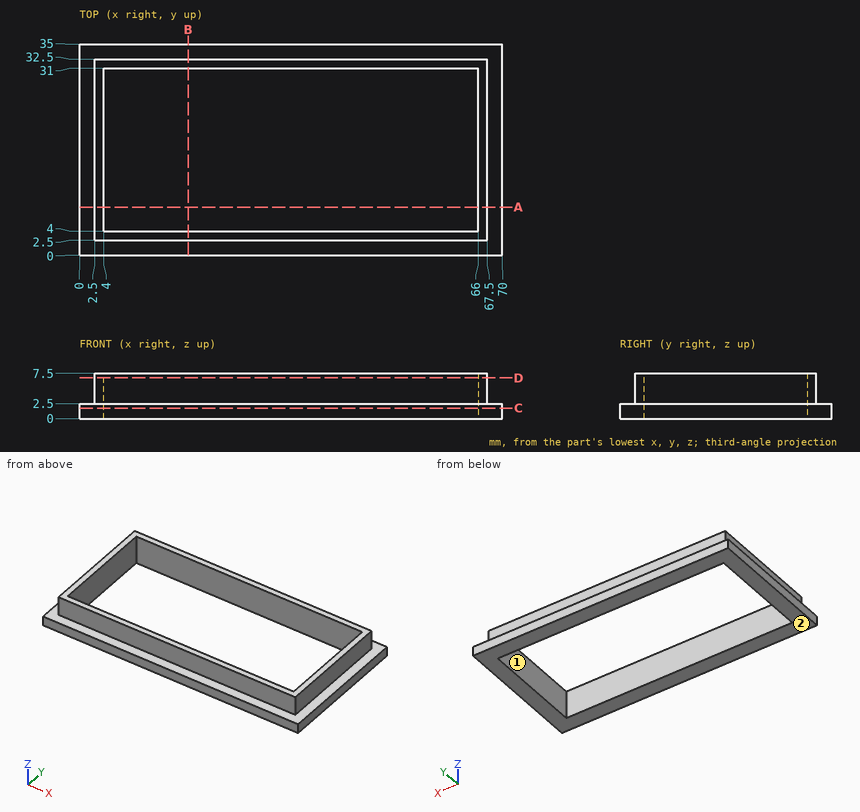
The drawing under review shows one solid part. Ordinate dimensions are in mm from its lowest x, y, z. Coordinates: 2 decimals unless noted, no trailing zeros. Write each loop counter-clockwise with the first axis right and the second up, starting at its lowest first coordinate (ties: lowest second). Pieces come first, ordered by that corner, then holes. Notation, with made-up numbers: M 15.25,-15.75 L 66.25,-15.75 A26 ccw 66.25,4.25 Z; hole C 3,78 d4. An arc over 180 degrees is marked long. Put each result on its own line as item: value.
1) Add section D-D on z = 6.75. Give the boundary of the cut face in (x, y), then the cut area to 3 significant figures.
Computed:
outline: M 2.5,2.5 L 67.5,2.5 L 67.5,32.5 L 2.5,32.5 Z; hole M 4,4 L 66,4 L 66,31 L 4,31 Z
area: 276 mm2
2) Wall thickness on probe 1 along Y at (x, z) = (34.5, 0.5); probe 2 along X at (y, z) = (16, 6.75); probe 3 along X at (y, z) = (15.5, 0.75): over which ranges is each line inside the solid? List them lowest first. Write a range as [from, to].
Computed:
probe 1: y = [0, 4], [31, 35]
probe 2: x = [2.5, 4], [66, 67.5]
probe 3: x = [0, 4], [66, 70]
3) Add section B-B on x = 18. Give the boundary of the cut face in (y, z), then the cut area to 3 significant figures.
Computed:
outline: M 0,0 L 4,0 L 4,7.5 L 2.5,7.5 L 2.5,2.5 L 0,2.5 Z; M 31,0 L 35,0 L 35,2.5 L 32.5,2.5 L 32.5,7.5 L 31,7.5 Z
area: 35.0 mm2
4) Add section C-C on z = 1.75. Give the boundary of the cut face in (x, y).
Computed:
outline: M 0,0 L 70,0 L 70,35 L 0,35 Z; hole M 4,4 L 66,4 L 66,31 L 4,31 Z
5) Add section A-A on y = 8. Give the boundary of the cut face in (x, z).
Computed:
outline: M 0,0 L 4,0 L 4,7.5 L 2.5,7.5 L 2.5,2.5 L 0,2.5 Z; M 66,0 L 70,0 L 70,2.5 L 67.5,2.5 L 67.5,7.5 L 66,7.5 Z
6) Draft analysis for pull direction X (two halves, no side actions). For the marked faces 1 and 2, state which applies: released by +X, released by -X, zero draft, split by the parting line, or undercut.
Computed:
face 1: undercut
face 2: zero draft
7) Clearance check with flat-ended pins moving along their axes: pin 1 Ø4 at (x, y) = (8.5, 7.5) entering from +Z; pin 2 Ø1.5 at (y, z) = (10.5, 4) entering from -X; pin 3 Ø1.5 at (x, z) = (45, 4.5) entering from -Y; pin 4 Ø3 at (x, z) = (44.5, 5) entering from +Y. State where each tip first meets the part, or that it passes through.
Computed:
pin 1: passes through
pin 2: stops at x = 2.5
pin 3: stops at y = 2.5
pin 4: stops at y = 32.5
